```python
from build123d import *
from build123d import SkipClean  # not in build123d's __all__

# Parameters (mm, degrees)
F0_R      = 12.5
F0_R_2    = 7.5
F1_DEPTH  = 64
F2_R      = 38.1
F2_R_2    = 25
F3_DEPTH  = 100
F4_DEPTH  = 50
F5_SIZE   = 3
F6_R      = 25
F7_DEPTH  = 200
F8_R      = 7.5
F9_DEPTH  = 50
F10_DEPTH = 100
F11_R     = 7.5
F12_DEPTH = 50
F13_DEPTH = 250


with BuildPart() as f1:
    # F0 (on Front) → F1 (new body)
    with BuildSketch(Plane.XZ):
        Circle(F0_R)
        Circle(F0_R_2, mode=Mode.SUBTRACT)
    extrude(amount=F1_DEPTH)

    # F2 (on Right) → F3 (join)
    with BuildSketch(Plane.YZ):
        Circle(F2_R)
        Circle(F2_R_2, mode=Mode.SUBTRACT)
    extrude(amount=F3_DEPTH)

    # F2 (on Right) → F4 (join)
    with BuildSketch(Plane.YZ):
        Circle(F2_R)
        Circle(F2_R_2, mode=Mode.SUBTRACT)
    extrude(amount=-F4_DEPTH)

    # F5
    f5_edges = [f1.edges().sort_by_distance(p)[0] for p in [
        (-12.5, -64, 0),
    ]]
    chamfer(f5_edges, length=F5_SIZE)

    # F6 (on face) → F7 (cut)
    with BuildSketch(Plane(origin=(-50, 0, 0), x_dir=(0, -1, 0), z_dir=(-1, 0, 0))):
        Circle(F6_R)
    extrude(amount=-F7_DEPTH, mode=Mode.SUBTRACT)

    # F8 (on face) → F9 (cut)
    with BuildSketch(Plane.XZ.offset(64)):
        Circle(F8_R)
    extrude(amount=-F9_DEPTH, mode=Mode.SUBTRACT)

    # F10 (add): a face of the model
    f10_faces = [f1.faces().sort_by_distance(p)[0] for p in [
        (100, -37.0223692655, 0),
    ]]
    with SkipClean():  # cleaning this boolean's faces spoils the solid; the shape is the same uncleaned
        extrude(f10_faces, amount=F10_DEPTH)

    # F11 (on face) → F12 (cut)
    with BuildSketch(Plane.XZ.offset(64)):
        Circle(F11_R)
    with SkipClean():  # cleaning this boolean's faces spoils the solid; the shape is the same uncleaned
        extrude(amount=-F12_DEPTH, mode=Mode.SUBTRACT)

    # F13 (add): a face of the model
    f13_faces = [f1.faces().sort_by_distance(p)[0] for p in [
        (200, -37.0223692655, 0),
    ]]
    extrude(f13_faces, amount=F13_DEPTH)

    # F14 (on Top) → F15 (revolve, cut)
    with BuildSketch(Plane.XY):
        Polygon((455.1408666709, 52.4849742776), (427.6145875454, 51.9348941743), (427.6145875454, -50.6588555872), (455.1408666709, -51.4342445287), align=None)
    with SkipClean():  # cleaning this boolean's faces spoils the solid; the shape is the same uncleaned
        revolve(axis=Axis((478.6976158619, 0.4289562068, 0), (0, -1, 0)), mode=Mode.SUBTRACT)


solid = f1.part
```
Verification items for the finished model (mm, model axes). A direction names the side the tool comes from. Round coordinates to 2 decimals unless told otherwise and drop trailing zeros. Write each loop counter-clockwise with the first axis right and the second up, starting at its lowest first coordinate (ties: lowest second). Pieces come first, ordered by that corner, then holes. Notation, with made-up numbers: (-36, -14.5) - (-27, -14.5) arc R10 cw to (-27, -0.5) - close; hole circle Ø5 at (23.25, 81.5). An arc over 180 degrees is marked (long way). Answer as a JSON object with one key per item and string values. Group by question number.
Q1. Go/stop test with flat-tipped pins: pin 1 Ø1.5 at (x, y) = (163, 3) entering from -Z; pin 2 Ø10 at (x, y) = (329, -29) entering from +Z; pin 3 Ø12 at (y, z) = (8, 24) entering from +X. Record where each tip stops, or that it passes through.
Q2. Section check C-C, the plane x = 225. Enter the section's corners in (y, z).
Q3. Section check A-A, the plane y = 0. Enter the section's corners in (x, z), plus the area to 3 significant figures.
Q4. Thickness scan on line 1 (X direction, y = -28.75, z = 0); line 2 (Z direction, x = 328, y = 0); line 3 (Z direction, x = 0, y = -52). Record the ranges inside material, lowest first.
Q5. Tool access check on faces 1 (the flat face through (-50, 8, -25)), 2 (the cylindrical face through (-1.627, -48.32, 12.394)). Record the directions out of +Z, -Z, +X, -X, +Y, -Y that give a thin tool (end or side, any length) a straight path to the whole face; none if there is none.
Q6. Section check B-B, the plane z = -18.5. Enter the section's corners in (x, y), plus the area to 3 significant figures.
Found:
{
 "1": {"pin 1": "stops at z = -38.03", "pin 2": "stops at z = 29.59", "pin 3": "stops at x = 437.35"},
 "2": {"outline": "circle Ø76.2 at (0, 0); hole circle Ø50 at (0, 0)"},
 "3": {"outline": "(-50, -38.1) - (444.67, -38.1) arc R51.08 cw to (434.15, -25) - (-50, -25) - close; (-50, 25) - (434.15, 25) arc R51.08 cw to (444.67, 38.1) - (-50, 38.1) - close", "area": "12,800 mm^2"},
 "4": {"line 1": "x = -50 to -7.5, 7.5 to 427.61", "line 2": "z = -38.1 to -25, 25 to 38.1", "line 3": "z = -12.5 to -7.5, 7.5 to 12.5"},
 "5": {"face 1": "+Z, -Z, -X, +Y, -Y", "face 2": "-Y"},
 "6": {"outline": "(-50, -33.31) - (431.08, -33.31) - (431.08, -16.82) - (-50, -16.82) - close; (-50, 16.82) - (431.08, 16.82) - (431.08, 33.31) - (-50, 33.31) - close", "area": "15,900 mm^2"}
}
